from build123d import *

# Parameters (mm, degrees)
BOSS_EXTRUDE1_DEPTH      = 15
BOSS_EXTRUDE1_DEPTH_BACK = 15
SKETCH1_W                = 76
SKETCH1_H                = 26
BOSS_EXTRUDE2_DEPTH      = 13
BOSS_EXTRUDE3_REACH      = 66.525
SKETCH3_W                = 13
SKETCH3_H                = 20
FILLET1_R                = 5
CHAMFER1_SIZE            = 1
SKETCH4_R                = 5
BOSS_EXTRUDE4_DEPTH      = 2


with BuildPart() as part:
    # Sketch1 → Boss-Extrude1 (new, two sides: drawn at the far end of the back side and taken through both)
    with BuildSketch(Plane(origin=(0, 0, 0), x_dir=(1, 0, 0), z_dir=(0, 1, 0)).offset(-BOSS_EXTRUDE1_DEPTH_BACK)):
        Rectangle(SKETCH1_W, SKETCH1_H)
    extrude(amount=BOSS_EXTRUDE1_DEPTH + BOSS_EXTRUDE1_DEPTH_BACK)

    # Sketch3 → Boss-Extrude3 (add, up to next)
    with BuildSketch(Plane(origin=(11.766324296, 0, 25.232963882), x_dir=(-0.9063077870366482, 0, 0.4226182617407034), z_dir=(-0.4226182617407034, 0, -0.9063077870366482)), mode=Mode.PRIVATE) as boss_extrude3_sk1:
        with Locations((-22.445658505, 0)):
            Rectangle(SKETCH3_W, SKETCH3_H)
    boss_extrude3_tool1 = extrude(boss_extrude3_sk1.sketch, amount=BOSS_EXTRUDE3_REACH, mode=Mode.PRIVATE) - part.part


with BuildPart() as body_2:
    # Sketch2 → Boss-Extrude2 (new body)
    with BuildSketch(Plane(origin=(26.233675704, 0, -12.232963882), x_dir=(0, 1, 0), z_dir=(-0.9063077870366482, 0, 0.42261826174070327))):
        with BuildLine():
            Line((10, -27.841495178), (-10, -27.841495178))
            Line((-10, -27.841495178), (-10, -47.841495178))
            ThreePointArc((-10, -47.841495178), (0, -57.841495178), (10, -47.841495178))
            Line((10, -47.841495178), (10, -27.841495178))
        make_face()
    extrude(amount=BOSS_EXTRUDE2_DEPTH)


with BuildPart() as part_1:
    add(part.part)

    add(body_2.part)  # Boss-Extrude3 merges body 2
    add(boss_extrude3_tool1.solids().sort_by_distance((32.108999, 0, 15.747019))[0])

    # Fillet1
    fillet1_edges = [part_1.edges().sort_by_distance(p)[0] for p in [
        (42.226182617, -10, 22.06307787),
        (50.678547852, 0, 40.189233611),
        (42.226182617, 10, 22.06307787),
    ]]
    fillet(fillet1_edges, radius=FILLET1_R)

    # Chamfer1
    chamfer1_edges = [part_1.edges().sort_by_distance(p)[0] for p in [
        (38, 15, 0),
        (-38, -15, 0),
        (0, 15, -13),
        (-38, 15, 0),
        (0, 15, 13),
        (0, -15, 13),
        (29.163225528, -10, 24.810096572),
        (29.163225528, 10, 24.810096572),
        (38.896546621, 0, 45.683271014),
        (38, -15, 0),
        (-38, 0, 13),
        (-38, 0, -13),
        (38, 0, -13),
        (0, -15, -13),
    ]]
    chamfer(chamfer1_edges, length=CHAMFER1_SIZE)

    # Sketch4 → Boss-Extrude4 (add)
    with BuildSketch(Plane(origin=(0, 15, 0), x_dir=(1, 0, 0), z_dir=(0, 1, 0))):
        with Locations(Location((-28, 0, 0), (0, 0, 270))):
            Circle(SKETCH4_R)
    extrude(amount=BOSS_EXTRUDE4_DEPTH)


solid = part_1.part
Geometry: final body of the model. Coordinates: model frame, mm. A direction names the side the tool comes from. Round coordinates to 2 decimals unless told otherwise and drop trailing zeros. Loops run counter-clockwise (first coordinate to the right, second up) from the corner with the lowest first, then second, coordinate; pieces in that order, holes last. Notation, with made-up numbers: (-10.75, 16) - (39.25, 16) arc R17 ccw to (39.25, 49) - close; hole circle Ø4 at (32.5, 19.25). An arc over 180 degrees is marked (long way). Write each question's results on one line, items separated by ' | '. Start each with the question number.
1) Cut plane B-B on z = 0. Return loops of the section in (x, y).
2) First-contact query: P1, Ø12, axis at y = 7, z = 29.5, coming from the -X side; P2, Ø6, axis at x = -3.5, y = 8, coming from the +Z side; P3, Ø19, axis at x = 30, z = 23.5, coming from the +Y side. Flat tips, straight axial feed; report the tip coordinate or a pass-through.
3) Mould query, pull axis Z, two halves, no side actions, for faces 6 (the face through (40.305, 8.574, 21.5)), 7 (the face through (43.21, -0.07, 24.17)), 8 (the face through (40.44, -8.57, 21.78)), 9 (the face through (29.687, -9.493, 24.767)). Classes: released by +Z, released by -Z, zero draft, split by the parting line, or undercut.
4) Line query: probe 1 along Z at (x, y) = (-12, 0.5); probe 2 along Y at (x, z) = (22.5, 9.5); probe 3 along X at (y, z) = (11, 11). Output: solid intervals per line, ascending. Write a range as [from, to].
5) Access query for faces 1 (the face through (33, -10, 23)), 2 (the face through (33, 10, 23)), 3 (the face through (38, 0, 1)), 4 (the face through (-32.88, 15.99, -1.08)), 5 (the face through (29.53, 9.49, 24.44)). Directions: +Z, -Z, +X, -X, +Y, -Y. A direction counts if a zero-diameter tool reaches every point of the face in a straight line with its end or side. Return the directions, or none.
6) Cut plane C-C on z = 8. Return loops of the section in (x, y).
7) Cut plane A-A on x = -12.5. Return loops of the section in (y, z).
8) Cut plane D-D on x = -28. Return loops of the section in (y, z).
Verdict:
1) outline: (-38, -14) - (-37, -15) - (37, -15) - (38, -14) - (38, 14) - (37, 15) - (-23, 15) - (-23, 17) - (-33, 17) - (-33, 15) - (-37, 15) - (-38, 14) - close
2) P1: stops at x = 28.55 | P2: stops at z = 13 | P3: stops at y = 10
3) face 6: undercut | face 7: released by -Z | face 8: undercut | face 9: released by +Z
4) probe 1: z = [-13, 13] | probe 2: y = [-15, 15] | probe 3: x = [-38, 38]
5) face 1: +Z, +X, -X, -Y | face 2: +Z, +X, -X, +Y | face 3: -Z, +X, +Y, -Y | face 4: +Y | face 5: +Z, -X, +Y
6) outline: (-38, -14) - (-37, -15) - (37, -15) - (38, -14) - (38, 14) - (37, 15) - (-37, 15) - (-38, 14) - close
7) outline: (-15, -12) - (-14, -13) - (14, -13) - (15, -12) - (15, 12) - (14, 13) - (-14, 13) - (-15, 12) - close
8) outline: (-15, -12) - (-14, -13) - (14, -13) - (15, -12) - (15, -5) - (17, -5) - (17, 5) - (15, 5) - (15, 12) - (14, 13) - (-14, 13) - (-15, 12) - close
